CAD build for the part. Positions are in the model's coordinates, mm. Face numbers are marked on the shaded views. A direction names the side the tool comes from. Coordinates: 2 decimals unless noted, no trailing zeros. Order: outer loops, then holes, each group sorted by start corner. A loop starts at its lowest first (then second) coordinate and runs counter-clockwise, first axis right, second up. Notation, with made-up numbers: (54.25, -17) - (110.25, -17) arc R9 ccw to (110.25, -5) - close; hole circle Ø3 at (0, 57). An arc over 180 degrees is marked (long way). Use one line per item in the form item = value.
```python
from build123d import *

# Parameters (mm, degrees)
F0_W     = 17
F0_H     = 20
F1_DEPTH = 1.2
F3_DEPTH = 8.5
F5_DEPTH = 8.5


with BuildPart() as f1:
    # F0 (on Top) → F1 (new body)
    with BuildSketch(Plane.XY):
        Rectangle(F0_W, F0_H)
    extrude(amount=F1_DEPTH)

    # F2 (on Right) → F3 (join, symmetric)
    with BuildSketch(Plane.YZ):
        Polygon((-10, 1.2), (-8.4, 1.2), (-8.4, 2.4), align=None)
    extrude(amount=F3_DEPTH, both=True)

    # F4 (on Right) → F5 (join, symmetric)
    with BuildSketch(Plane.YZ):
        Polygon((10, 1.2), (10, 0), (10, -3), (-10, -3), (-10, -4.6), (16, -4.6), (16, -3), align=None)
    extrude(amount=F5_DEPTH, both=True)


solid = f1.part
```
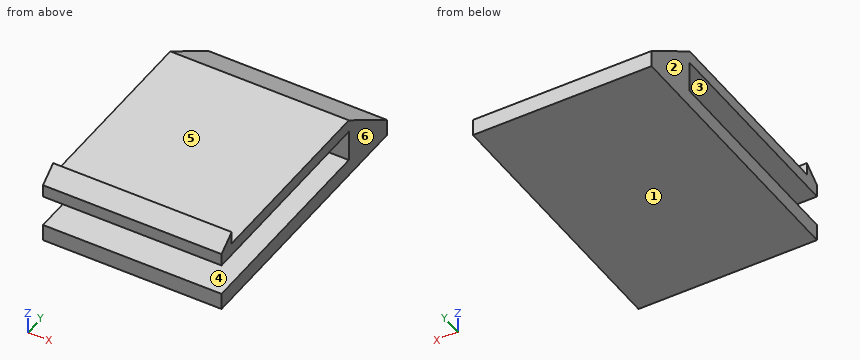
Item 1: Cut at D-D, the plane y = 10.5. Write the cut outline in (x, z).
Derived:
outline = (-8.5, -4.6) - (8.5, -4.6) - (8.5, 0.85) - (-8.5, 0.85) - close
Item 2: Cut at C-C, the plane z = 1.5. Write the cut outline in (x, y), plus the area to 3 significant figures.
Derived:
outline = (-8.5, -9.6) - (8.5, -9.6) - (8.5, -8.4) - (-8.5, -8.4) - close
area = 20.4 mm²
Item 3: Cut at A-A, the plane y = 5. Write the cut outline in (x, z).
Derived:
outline = (-8.5, -4.6) - (8.5, -4.6) - (8.5, -3) - (-8.5, -3) - close; (-8.5, 0) - (8.5, 0) - (8.5, 1.2) - (-8.5, 1.2) - close
Item 4: Drop flat-ended pins along their axis: pin 1 (1.3 mm diameter, centred on x = 2, z = 2, fed in from +Y); pin 2 (2 mm diameter, centred on x = 6.5, z = -1.5, fed in from -Y); pin 3 (4 mm diameter, centred on x = 1, y = 6.5, fed in from +Z). Give the stop position or say it passes through.
Derived:
pin_1 = -8.4
pin_2 = 10
pin_3 = 1.2
Item 5: Two-plate mould, pull along Z, no slides. Class the marked faces 1, 2 and 3: +Z half, -Z half, draft (parallel to the pull), parting line (faces both ways), or undercut.
Derived:
face_1 = -Z half
face_2 = draft
face_3 = undercut
Item 6: Cut at B-B, the plane x = -3.5. Write the cut outline in (y, z).
Derived:
outline = (-10, -4.6) - (16, -4.6) - (16, -3) - (10, 1.2) - (-8.4, 1.2) - (-8.4, 2.4) - (-10, 1.2) - (-10, 0) - (10, 0) - (10, -3) - (-10, -3) - close
Item 7: Drill centre lines: line 1 (Z direction, x = -6, y = -8); line 2 (Z direction, x = -4.5, y = 11.5); line 3 (Y direction, x = 7, z = 1.75). Where is each one in solid material? Low to high. Write a range as [from, to].
Derived:
line_1 = [-4.6, -3], [0, 1.2]
line_2 = [-4.6, 0.15]
line_3 = [-9.27, -8.4]
Item 8: 3-axis set-ups, long thin cutter, end or side, ignore diameter. For the marked faces 4, 5 and 6: which of +Z, -Z, +X, -X, +Y, -Y reach the whole face in a straight line?
Derived:
face_4 = +X, -X, -Y
face_5 = +Z, +X, -X, +Y
face_6 = +Z, -Z, +X, +Y, -Y
